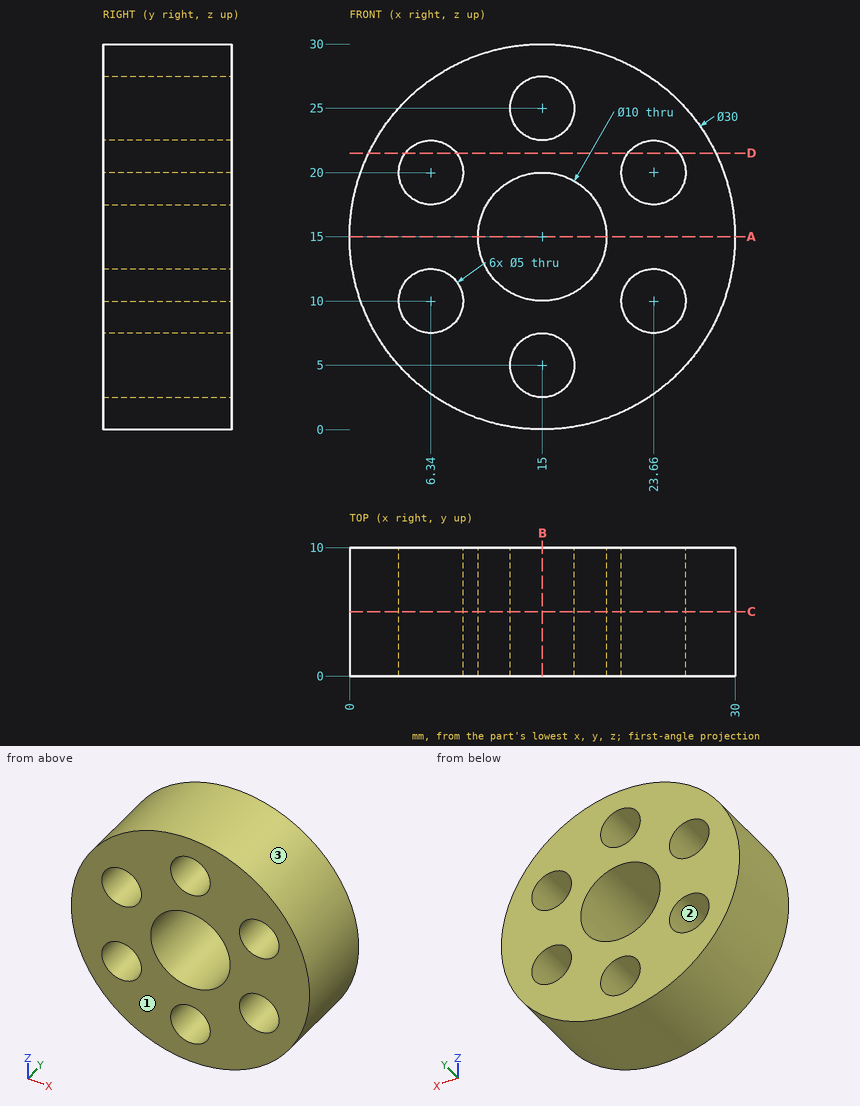
Check sheet for the drawn part. Datum: minimum x, y, z corner. Units: mm. Give positions to 0.01 mm unless a question says otherwise; leave off trailing zeros. Loops run counter-clockwise (first coordinate to the right, second up) from the corner with the lowest first, then second, coordinate; pieces in that order, holes last.
1) Thickness scan on line 1 along X through (y, z) = (2.75, 12); line 2 along Z through (x, y) = (23.75, 5.75); line 3 along Z through (x, y) = (15.25, 7.5). Record the ranges inside material, lowest first.
2) Sectioned sample at B-B, the plane x = 15. Enter the section's corners in (y, z), then the cut area to 3 significant figures.
3) Depth check by flat-ended pin: pin 1 Ø4 at (x, z) = (6.34, 10) entering from +Y; pin 2 Ø4 at (y, z) = (2.5, 17.5) entering from -X; pin 3 Ø3 at (y, z) = (9, 9) entering from +X; pin 4 Ø2 at (x, y) = (19, 7) entering from -Z. Enter the tip coordinate at first touch or a pass-through.
4) Sectioned sample at A-A, the plane z = 15. Enter the section's corners in (x, y), then the cut area to 3 significant figures.
5) Sectioned sample at C-C, the plane y = 5. Count the separate pieces of the cut face and the enclosed holes in it.
6) Sectioned sample at D-D, the plane z = 21.5. Enter the section's corners in (x, y).
7) Draft check along Z on the marked faces 1, 2 and 3. Enter one of: pulls with the +Z half, pulls with the -Z half, needs draft (parallel to the pull), parting line crosses it, or undercut.
Answers:
1. line 1: x = 0.3 to 4.84, 7.84 to 11, 19 to 22.16, 25.16 to 29.7
1. line 2: z = 2.82 to 7.5, 12.5 to 17.5, 22.5 to 27.18
1. line 3: z = 0 to 2.51, 7.49 to 10.01, 19.99 to 22.51, 27.49 to 30
2. outline: (0, 0) - (10, 0) - (10, 2.5) - (0, 2.5) - close; (0, 7.5) - (10, 7.5) - (10, 10) - (0, 10) - close; (0, 20) - (10, 20) - (10, 22.5) - (0, 22.5) - close; (0, 27.5) - (10, 27.5) - (10, 30) - (0, 30) - close
2. area: 100 mm2
3. pin 1: passes through
3. pin 2: stops at x = 0.01
3. pin 3: stops at x = 29.31
3. pin 4: stops at z = 0.3
4. outline: (0, 0) - (10, 0) - (10, 10) - (0, 10) - close; (20, 0) - (30, 0) - (30, 10) - (20, 10) - close
4. area: 200 mm2
5. separate pieces: 1
5. enclosed holes: 7
6. outline: (1.48, 0) - (4.34, 0) - (4.34, 10) - (1.48, 10) - close; (8.34, 0) - (21.66, 0) - (21.66, 10) - (8.34, 10) - close; (25.66, 0) - (28.52, 0) - (28.52, 10) - (25.66, 10) - close
7. face 1: needs draft
7. face 2: undercut
7. face 3: parting line crosses it
